from build123d import *

# Parameters (mm, degrees)
F2_R     = 19.0246
F3_DEPTH = 53.849
F4_R     = 6.35
F5_DEPTH = 19.051
F6_R     = 3.048


# Not quite as in the source:
# - a feature names something its author has since deleted; it is built from what else it names


with BuildPart() as f1:
    # F0 (on Right) → F1 (revolve)
    with BuildSketch(Plane.YZ):
        Polygon((0, 34.925), (0, 0), (53.848, 0), (53.848, 69.85), (34.798, 69.85), (34.798, 34.925), align=None)
    revolve(axis=Axis((0, 26.924, 0), (0, 1, 0)))

    # F2 (on face) → F3 (cut, through all)
    with BuildSketch(Plane.XZ):
        Circle(F2_R)
    extrude(amount=-F3_DEPTH, mode=Mode.SUBTRACT)

    # F4 (on face) → F5 (cut, through all)
    with BuildSketch(Plane.XZ.offset(-34.798)):
        with Locations((0, 53.848)):
            Circle(F4_R)
        with Locations((-53.848, 0)):
            Circle(F4_R)
        with Locations((53.848, 0)):
            Circle(F4_R)
        with Locations((0, -53.848)):
            Circle(F4_R)
    extrude(amount=-F5_DEPTH, mode=Mode.SUBTRACT)

    # F6
    f6_edges = [f1.edges().sort_by_distance(p)[0] for p in [
        (0, 34.798, -34.925),
        (0, 0, -34.925),
        (0, 34.798, -69.85),
    ]]
    fillet(f6_edges, radius=F6_R)


solid = f1.part
Build history of the part. All positions in model axes, mm. A direction names the side the tool comes from. Round coordinates to 2 decimals unless told otherwise and drop trailing zeros. Order: outer loops, then holes, each group sorted by start corner. A loop starts at its lowest first (then second) coordinate and runs counter-clockwise, first axis right, second up. Notation, with made-up numbers: M 32.25,-31.75 L 60.25,-31.75 A28 cw 60.25,-4.75 Z; hole C 83,-2 d9. An arc over 180 degrees is marked long. Use CSV: the item, a comma, the result in double quotes. Start each with the question number.
(1) Cut at D-D on y = 43. List the corners of the cut face in (x, z).
(2) Drill centre lines: probe 1 along Y at (x, z) = (18.5, -55); probe 2 along Z at (x, y) = (-17, 10); probe 3 along X at (y, z) = (23, 14.5). Where is each one in solid material? Low to high.
(3) Cut at C-C on y = 22.5. List the corners of the cut face in (x, z) (3 decimals), then the cut area to 3 significant figures.
(4) Mould opens along X. For faces 1 (the face through (-60.19, 44.19, 0.28)), 2 (the face through (-14, 0, 14)), 3 (the face through (-21.251, 17.198, -27.715)) say: +X half, -X half, draft (parallel to the pull), parting line (faces both ways), or undercut.
(5) Cut at A-A on z = 0. List the corners of the cut face in (x, y) (3 decimals).
(6) Cut at B-B on x = 0. List the corners of the cut face in (y, z) (3 decimals).
(7) Tool access for faces 4 (the face through (-29, 34.798, 29)), 5 (the face through (-15, 53.848, -15)): list every direction of +Z, -Z, +X, -X, +Y, -Y with a clear straight run to the whole face (end or side of a thin tool).
(8) Flat gauge pins, fed straight in: P1, Ø16.5, axis at x = 0, z = 53.848, coming from the -Y side; P2, Ø10, axis at x = 28, y = 43.5, coming from the +Z side; P3, Ø12, axis at x = 2.5, y = 26.5, coming from the -Z side. Where does each tip first touch, or does it go through?
Findings:
1,outline,"C 0,0 d139.7; hole C -53.85,0 d12.7; hole C 0,0 d38.05; hole C 0,-53.85 d12.7; hole C 0,53.85 d12.7; hole C 53.85,0 d12.7"
2,probe 1,"y = 34.8 to 53.85"
2,probe 2,"z = -30.51 to -8.54, 8.54 to 30.51"
2,probe 3,"x = -31.77 to -12.32, 12.32 to 31.77"
3,outline,"C 0,0 d69.85; hole C 0,0 d38.049"
3,area,"2,690 mm^2"
4,face 1,"undercut"
4,face 2,"draft"
4,face 3,"parting line"
5,outline,"M -69.85,37.846 A3.048 ccw -66.802,34.798 L -60.198,34.798 L -60.198,53.848 L -69.85,53.848 Z; M -47.498,34.798 L -37.973,34.798 A3.048 cw -34.925,31.75 L -34.925,3.048 A3.048 ccw -31.877,0 L -19.025,0 L -19.025,53.848 L -47.498,53.848 Z; M 19.025,0 L 31.877,0 A3.048 ccw 34.925,3.048 L 34.925,31.75 A3.048 cw 37.973,34.798 L 47.498,34.798 L 47.498,53.848 L 19.025,53.848 Z; M 60.198,34.798 L 66.802,34.798 A3.048 ccw 69.85,37.846 L 69.85,53.848 L 60.198,53.848 Z"
6,outline,"M 0,-31.877 A3.048 ccw 3.048,-34.925 L 31.75,-34.925 A3.048 cw 34.798,-37.973 L 34.798,-47.498 L 53.848,-47.498 L 53.848,-19.025 L 0,-19.025 Z; M 0,19.025 L 53.848,19.025 L 53.848,47.498 L 34.798,47.498 L 34.798,37.973 A3.048 cw 31.75,34.925 L 3.048,34.925 A3.048 ccw 0,31.877 Z; M 34.798,-66.802 A3.048 ccw 37.846,-69.85 L 53.848,-69.85 L 53.848,-60.198 L 34.798,-60.198 Z; M 34.798,60.198 L 53.848,60.198 L 53.848,69.85 L 37.846,69.85 A3.048 ccw 34.798,66.802 Z"
7,face 4,"-Y"
7,face 5,"+Z, -Z, +X, -X, +Y"
8,P1,"stops at y = 34.8"
8,P2,"stops at z = 65.95"
8,P3,"stops at z = -34.97"
